from build123d import *

# Parameters (mm, degrees)
F4_D           = 3.5
F4_DEPTH       = 11.5
F4_TIP         = 1.0515060833
F4_ON_F2_D     = 3.5
F4_ON_F2_DEPTH = 11.5
F4_ON_F2_TIP   = 1.0515060833


with BuildPart() as f1:
    # F0 (on Front) → F1 (revolve)
    with BuildSketch(Plane.XZ):
        Polygon((53, 4), (43, 4), (-43, 4), (-53, 4), (-53, 3), (-93, 3), (-93, 0), (93, 0), (93, 3), (53, 3), align=None)
    revolve(axis=Axis((0, 0, 0), (-1, 0, 0)))

    # F4
    with Locations(Plane.YZ.offset(93)):
        with Locations((0, 0)):
            Hole(F4_D / 2, depth=F4_DEPTH)
            with Locations((0, 0, -(F4_DEPTH + F4_TIP / 2))):  # 118° drill point
                Cone(0, F4_D / 2, F4_TIP, mode=Mode.SUBTRACT)

    # F4 on F2
    with Locations(Plane(origin=(-93, 0, 0), x_dir=(0, -1, 0), z_dir=(-1, 0, 0))):
        with Locations((0, 0)):
            Hole(F4_ON_F2_D / 2, depth=F4_ON_F2_DEPTH)
            with Locations((0, 0, -(F4_ON_F2_DEPTH + F4_ON_F2_TIP / 2))):  # 118° drill point
                Cone(0, F4_ON_F2_D / 2, F4_ON_F2_TIP, mode=Mode.SUBTRACT)


solid = f1.part
Verification items for the finished model (mm, model axes). A direction names the side the tool comes from. Coordinates: 2 decimals unless noted, no trailing zeros. Order: outer loops, then holes, each group sorted by start corner. A loop starts at its lowest first (then second) coordinate and runs counter-clockwise, first axis right, second up. Notation, with made-up numbers: (12, 68) -> (18, 68) arc R33 ccw to (18, 107) -> close; hole circle Ø5 at (49, 53.25). An arc over 180 degrees is marked (long way). Put each result on its own line as item: value. Start each with the question number.
1. Go/stop test with flat-tipped pins: pin 1 Ø2 at (x, z) = (-33, -2) entering from -Y; pin 2 Ø2 at (y, z) = (0, 0) entering from -X; pin 3 Ø1.5 at (x, y) = (-28, -2) entering from +Z. Record where each tip stops, or that it passes through.
2. Mould release check, pull along Z, two halves, no side actions. Record for faces 4 (the conical face through (-80.631, 0.066, -0.297)), 5 (the cylindrical face through (-0.742, -3.905, -0.867)), 6 (the cylindrical face through (87.17, -1.617, -0.67)), 7 (the flat face through (93, -2, 0)): released by +Z, released by -Z, zero draft, split by the parting line, or undercut.
3. Access from +Z, -Z, +X, -X, +Y, -Y to the whole of each face (thin tool, end or side, straight path). Record for faces 1 (the cylindrical face through (73, 0, -3)), 2 (the flat face through (-53, 3, 1)), 3 (the flat face through (-93, -2, 0)).
4. Material ranges on L1, parallel to Y at x = -84.5, z = 0; L2, parallel to X at y = -2.75, z = -1.5; L3, parallel to Z at x = -33, y = 0.25, recorded low to high. Write a range as [from, to].
5. Cross-section at A-A, the plane x = -46.5. Record the boundary of the cut face in (y, z), then the cut area to 3 significant figures.
Computed:
1. pin 1: y = -3.87
1. pin 2: x = -81.05
1. pin 3: z = 3.8
2. face 4: undercut
2. face 5: split by the parting line
2. face 6: undercut
2. face 7: zero draft
3. face 1: +X
3. face 2: -X
3. face 3: +Z, -Z, -X, +Y, -Y
4. L1: [-3, -1.75], [1.75, 3]
4. L2: [-53, 53]
4. L3: [-3.99, 3.99]
5. outline: circle Ø8 at (0, 0)
5. area: 50.3 mm2
